The model under review builds one solid part; all positions refer to its coordinate system, in mm. A direction names the side the tool comes from. Coordinates: 2 decimals unless noted, no trailing zeros. Write each loop counter-clockwise with the first axis right and the second up, starting at its lowest first coordinate (ties: lowest second). Pieces come first, ordered by that corner, then holes.
1) Add section B-B, the plane x = 0. State the section outline as (y, z) points, then the cut area to 3 significant figures.
2) Add section C-C, the plane y = -19.75. State the section outline as (x, z) points, then the cut area to 3 significant figures.
3) Add section A-A, the plane z = 1.05. Give the number of separate pieces and of enclosed holes in the cut face, then the cut area to 3 significant figures.
4) For line 1 (Y direction, x = 0, z = 1.5); line 2 (Y direction, x = 8, z = 1); line 3 (Y direction, x = 14, z = 1.1), list the stretches that pass through material, from the lowest coordinate up.
5) Machinability: for faces 4 (the cylindrical face through (21.37, -23.48, 0.99)), 5 (the flat face through (5, -25, 1)), which of the approach directions +Z, -Z, +X, -X, +Y, -Y give a long, thin tool a straight path to every point of the face, cutting with its end or side? Answer none if there is none.
6) For P1, Ø3, axis at x = -11.5, y = -25, coming from the +Z side; P2, Ø1, axis at y = -24, z = 1, coming from the +X side, all flat-tipped, find the tip position at first contact; note any pin that passes through.
7) Add section D-D, the plane y = -25.35. State the section outline as (x, z) points, then the cut area to 3 significant figures.
8) Mouldability with a two-part tool opening along Y and no side actions: class faces 1 (the flat face through (20.354, -13.837, 0.986)), 2 (the cylindrical face through (18.289, -8.866, 1.014)), 3 (the cylindrical face through (-21.48, -23.21, 0.99)) as released by +Y, released by -Y, zero draft, split by the parting line, or undercut.
from build123d import *

# Parameters (mm, degrees)
SKETCH1_R           = 0.9999999999999973
BOSS_EXTRUDE1_DEPTH = 2
BOSS_EXTRUDE2_DEPTH = 2
BOSS_EXTRUDE3_DEPTH = 2
BOSS_EXTRUDE4_DEPTH = 2
BOSS_EXTRUDE6_DEPTH = 2
CUT_EXTRUDE5_DEPTH  = 10
CUT_EXTRUDE6_DEPTH  = 10
FILLET3_R           = 10
FILLET4_R           = 15


with BuildPart() as part:
    # Sketch1 → Boss-Extrude1 (new body)
    with BuildSketch(Plane.XY):
        with BuildLine():
            Line((-25.026699742262835, -12.489403509000002), (-31.579999999831756, -12.489403509000002))
            ThreePointArc((-31.579999999831788, -12.489403509000118), (-4.3876e-13, -33.96), (31.579999999831465, -12.489403509000935))
            Line((31.579999999831173, -12.489403509000002), (25.026699742262835, -12.489403509000002))
            ThreePointArc((25.026699742262835, -12.489403508999999), (16.78917371704707, -22.3706179149977), (5.000000000000879, -27.51946402094327))
            Line((5.000000000000001, -27.519464020943122), (5.000000000000001, -21.97))
            Line((5.000000000000001, -21.97), (0, -21.97))
            Line((0, -21.97), (-5.000000000000001, -21.970000000000002))
            Line((-5.000000000000001, -21.970000000000002), (-5.000000000000001, -27.519464020943126))
            ThreePointArc((-5.000000000000872, -27.519464020943275), (-16.789173717047063, -22.370617914997695), (-25.02669974226283, -12.489403508999999))
        make_face()
        with Locations((2.25e-15, -25.35)):
            Circle(SKETCH1_R, mode=Mode.SUBTRACT)
    extrude(amount=BOSS_EXTRUDE1_DEPTH)

    # Sketch2 → Boss-Extrude2 (add)
    with BuildSketch(Plane.XY.offset(2)):
        with BuildLine():
            Line((-31.57999999983184, -12.489403509000002), (-25.026699742262828, -12.489403509000002))
            Line((-25.026699742262828, -12.489403509000002), (0, -12.489403509000002))
            Line((0, -12.489403509000002), (25.026699742262828, -12.489403509000002))
            Line((25.026699742262828, -12.489403509000002), (31.57999999983184, -12.489403509000002))
            ThreePointArc((31.57999999983184, -12.489403509000002), (30.972585231224635, -9.734010611787788), (29.262941504232284, -7.489403509000002))
            Line((29.262941504232288, -7.489403509000003), (-29.262941504232284, -7.489403509000003))
            ThreePointArc((-29.262941504232284, -7.489403509000002), (-30.972585231224635, -9.734010611787788), (-31.57999999983184, -12.489403509000002))
        make_face()
    extrude(amount=-BOSS_EXTRUDE2_DEPTH)

    # Sketch3 → Boss-Extrude3 (add)
    with BuildSketch(Plane.XY.offset(2)):
        Polygon((-24.813781653352383, -19.23578932070869), (-5, -19.235789320708687), (-5.000000000000001, -19.223614188291315), (25.52831463289919, -19.223614188291315), (25.52831463289919, -15.223614188291313), (4.937516262759692, -15.223614188291313), (4.937516262759691, -15.235789320708687), (-24.813781653352386, -15.235789320708694), align=None)
    extrude(amount=-BOSS_EXTRUDE3_DEPTH)

    # Sketch4 → Boss-Extrude4 (add)
    with BuildSketch(Plane.XY):
        Polygon((26.752232503098107, -20.918882764148314), (23.464067657719866, -15.223614188291315), (21.15466658096137, -15.223614188291313), (25.020181695529228, -21.918882764148307), align=None)
        Polygon((21.15466658096137, -15.223614188291313), (23.464067657719863, -15.223614188291313), (18.99871904006177, -7.489403509000002), (17.266668232492894, -8.489403508999997), align=None)
    extrude(amount=BOSS_EXTRUDE4_DEPTH)

    # Sketch6 → Boss-Extrude6 (add)
    with BuildSketch(Plane(origin=(0, 0, 0), x_dir=(-1, 0, 0), z_dir=(0, 0, -1))):
        Polygon((21.146762799182063, -15.235789320708694), (23.45616387594056, -15.235789320708694), (22.962540836382626, -14.38080913640776), (21.870537288251985, -12.489403509), (19.561136211493483, -12.489403509000002), align=None)
    extrude(amount=-BOSS_EXTRUDE6_DEPTH)

    # Sketch7 → Cut-Extrude5 (cut)
    with BuildSketch(Plane(origin=(0, 0, 0), x_dir=(-1, 0, 0), z_dir=(0, 0, -1))):
        with BuildLine():
            Line((23.456163875940437, -15.235789320708776), (26.743640561861312, -20.92986596942182))
            ThreePointArc((26.743640561861444, -20.929865969421787), (29.465608999795766, -16.88370475550775), (31.579999999831838, -12.489403509000006))
            ThreePointArc((31.579999999831834, -12.489403508999994), (30.972585231224627, -9.734010611787786), (29.262941504232284, -7.489403509000004))
            Line((29.262941504232284, -7.489403509000003), (18.983785942303626, -7.489403509000003))
            Line((18.98378594230363, -7.4894035090000095), (21.87053728825184, -12.489403509000091))
            Line((21.87053728825199, -12.489403509000002), (25.026699742262828, -12.489403509000002))
            ThreePointArc((25.02669974226283, -12.489403509000006), (24.280293962635962, -13.884819951586834), (23.456163875940568, -15.235789320708696))
        make_face()
    extrude(amount=-CUT_EXTRUDE5_DEPTH, mode=Mode.SUBTRACT)

    # Sketch8 → Cut-Extrude6 (cut)
    with BuildSketch(Plane(origin=(0, 0, 0), x_dir=(-1, 0, 0), z_dir=(0, 0, -1))):
        with BuildLine():
            Line((-26.752232503097716, -20.918882764147654), (-23.464067657719863, -15.223614188291315))
            ThreePointArc((-23.46406765771987, -15.223614188291315), (-24.283896058283027, -13.878519093567089), (-25.026699742262828, -12.489403509000002))
            Line((-25.026699742262828, -12.489403509000002), (-21.88547038600989, -12.489403509000002))
            Line((-21.88547038600989, -12.489403509000002), (-18.998719040061772, -7.4894035090000015))
            Line((-18.998719040061772, -7.489403509000003), (-29.262941504232288, -7.489403509000003))
            ThreePointArc((-29.262941504232284, -7.489403509000002), (-30.97258523122463, -9.73401061178779), (-31.57999999983184, -12.489403509000002))
            ThreePointArc((-31.57999999983184, -12.489403509000002), (-29.469074761896252, -16.877654833470505), (-26.75223250309883, -20.9188827641474))
        make_face()
    extrude(amount=-CUT_EXTRUDE6_DEPTH, mode=Mode.SUBTRACT)

    # Fillet3
    fillet3_edges = [part.edges().sort_by_distance(p)[0] for p in [
        (-18.983785942303626, -7.489403509000006, 1),
        (18.998719040061772, -7.489403509000002, 1),
    ]]
    fillet(fillet3_edges, radius=FILLET3_R)

    # Fillet4
    # the kernel refuses this fillet: 15 mm, written as the material it takes off along each edge
    with BuildSketch(Plane(origin=(26.752232503098277, -20.91888276414753, -41.15536178864485), x_dir=(-0.5000000000000459, 0.8660254037844121, 0), z_dir=(0, 0, 1))) as fillet4_piece_1:
        with BuildLine():
            CenterArc((12.63895144979885, 14.71592649800607), FILLET4_R, 173.92282911126543, 84.90866305824733)
            ThreePointArc((-2.2767516311276927, 16.30394463443854), (-2.1412465863768713, 8.011927210685023), (0, 0))
            Line((0, 0), (9.73352423417586, 7.4e-16))
        make_face()
    extrude(amount=84.3107235772897, mode=Mode.SUBTRACT)
    with BuildSketch(Plane(origin=(-26.743640561861376, -20.929865969421805, -41.183176669180206), x_dir=(0.7889080559016987, -0.6145112524058467, 0), z_dir=(0, 0, 1))) as fillet4_piece_2:
        with BuildLine():
            CenterArc((12.835180855907009, 14.552123643012767), FILLET4_R, 199.06172243650428, 84.97473929921648)
            Line((-1.342328727646797, 9.653325626331542), (0, 0))
            ThreePointArc((0, 0), (8.236635333836043, -1.0139920722190925), (16.473270667672082, 5.9e-16))
        make_face()
    extrude(amount=84.36635333836041, mode=Mode.SUBTRACT)


solid = part.part
Geometry results:
1. outline: (-33.96, 0) - (-26.35, 0) - (-26.35, 2) - (-33.96, 2) - close; (-24.35, 0) - (-21.97, 0) - (-21.97, 2) - (-24.35, 2) - close; (-19.22, 0) - (-15.24, 0) - (-15.24, 2) - (-19.22, 2) - close; (-12.49, 0) - (-7.49, 0) - (-7.49, 2) - (-12.49, 2) - close
1. area: 38.0 mm2
2. outline: (-22.48, 0) - (-19.81, 0) - (-19.81, 2) - (-22.48, 2) - close; (19.81, 0) - (22.49, 0) - (22.49, 2) - (19.81, 2) - close
2. area: 10.7 mm2
3. separate pieces: 1
3. enclosed holes: 3
3. area: 717 mm2
4. line 1: y = -33.96 to -26.35, -24.35 to -21.97, -19.22 to -15.24, -12.49 to -7.49
4. line 2: y = -33 to -26.8, -19.22 to -15.22, -12.49 to -7.49
4. line 3: y = -30.94 to -24.21, -19.22 to -15.22, -12.49 to -7.52
5. face 4: +Z, -Z, +X
5. face 5: +Z, -Z
6. P1: stops at z = 2
6. P2: stops at x = 21.36
7. outline: (-20.36, 0) - (-11.82, 0) - (-11.82, 2) - (-20.36, 2) - close; (-5, 0) - (-1, 0) - (-1, 2) - (-5, 2) - close; (1, 0) - (5, 0) - (5, 2) - (1, 2) - close; (11.82, 0) - (20.37, 0) - (20.37, 2) - (11.82, 2) - close
7. area: 50.2 mm2
8. face 1: undercut
8. face 2: released by +Y
8. face 3: split by the parting line
